The model under review builds one solid part; all positions refer to its coordinate system, in mm. Round coordinates to 2 decimals unless told otherwise and drop trailing zeros. Order: outer loops, then holes, each group sorted by start corner. A loop starts at its lowest first (then second) coordinate and runs counter-clockwise, first axis right, second up.
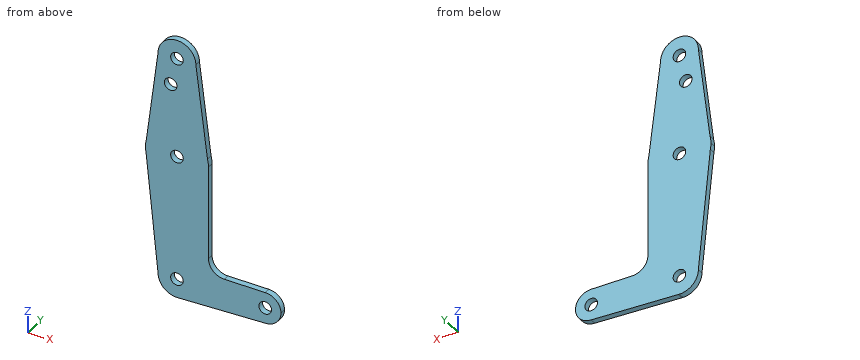
from build123d import *

# Parameters (mm, degrees)
F0_R     = 3.175
F1_DEPTH = 3.048


with BuildPart() as f1:
    # F0 (on Front) → F1 (new body)
    with BuildSketch(Plane.XZ):
        with BuildLine():
            ThreePointArc((-9.525, 114.3), (0, 104.775), (9.525, 114.3))
            ThreePointArc((9.525, 114.3), (0, 123.825), (-9.525, 114.3))
        make_face()
        with Locations((0, 114.3)):
            Circle(F0_R, mode=Mode.SUBTRACT)
        with BuildLine():
            Line((15.3865384615, 67.4076923077), (9.525, 114.3))
            ThreePointArc((9.525, 114.3), (0, 104.775), (-9.525, 114.3))
            Line((-9.525, 114.3), (-15.3865384615, 67.4076923077))
            ThreePointArc((-15.3865384615, 67.4076923077), (0, 79.375), (15.3865384615, 67.4076923077))
        make_face()
        with Locations((-3.175, 100.0252)):
            Circle(F0_R, mode=Mode.SUBTRACT)
        with BuildLine():
            Line((15.875, 63.5), (15.3865384615, 67.4076923077))
            ThreePointArc((15.3865384615, 67.4076923077), (0, 79.375), (-15.3865384615, 67.4076923077))
            Line((-15.3865384615, 67.4076923077), (-15.875, 63.5))
            Line((-15.875, 63.5), (-15.5606435644, 60.3564356436))
            ThreePointArc((-15.5606435644, 60.3564356436), (1.5796215395, 47.7037846054), (15.875, 63.5))
        make_face()
        with Locations((0, 63.5)):
            Circle(F0_R, mode=Mode.SUBTRACT)
        with BuildLine():
            ThreePointArc((15.875, 63.5), (15.7524112928, 65.4690514116), (15.3865384615, 67.4076923077))
            Line((15.3865384615, 67.4076923077), (15.875, 63.5))
        make_face()
        with BuildLine():
            Line((-15.875, 63.5), (-15.3865384615, 67.4076923077))
            ThreePointArc((-15.3865384615, 67.4076923077), (-15.7524112928, 65.4690514116), (-15.875, 63.5))
        make_face()
        with BuildLine():
            Line((15.875, 15.8877), (15.875, 63.5))
            ThreePointArc((15.875, 63.5), (1.5796215395, 47.7037846054), (-15.5606435644, 60.3564356436))
            Line((-15.5606435644, 60.3564356436), (-9.525, 0))
            ThreePointArc((-9.525, 0), (0, 9.525), (9.525, 0))
            ThreePointArc((9.525, 0), (6.9712901065, -6.4905114784), (0.6794904459, -9.5007324841))
            Line((0.6794904459, -9.5007324841), (44.45, -7.9375))
            ThreePointArc((44.45, -7.9375), (36.5125, 0), (44.45, 7.9375))
            Line((44.45, 7.9375), (23.8252, 7.9375))
            ThreePointArc((23.8252, 7.9375), (18.2035596682, 10.2660596682), (15.875, 15.8877))
        make_face()
        with BuildLine():
            Line((-15.5606435644, 60.3564356436), (-15.875, 63.5))
            ThreePointArc((-15.875, 63.5), (-15.7962153946, 61.9203784605), (-15.5606435644, 60.3564356436))
        make_face()
        with BuildLine():
            ThreePointArc((9.525, 0), (0, 9.525), (-9.525, 0))
            ThreePointArc((-9.525, 0), (-6.7351920908, -6.7351920908), (0, -9.525))
            Line((0, -9.525), (0.6794904459, -9.5007324841))
            ThreePointArc((0.6794904459, -9.5007324841), (6.9712901065, -6.4905114784), (9.525, 0))
        make_face()
        Circle(F0_R, mode=Mode.SUBTRACT)
        with BuildLine():
            Line((0.6794904459, -9.5007324841), (0, -9.525))
            ThreePointArc((0, -9.525), (0.3399618281, -9.5189311877), (0.6794904459, -9.5007324841))
        make_face()
        with BuildLine():
            ThreePointArc((52.3875, 0), (50.0626600757, 5.6126600757), (44.45, 7.9375))
            ThreePointArc((44.45, 7.9375), (36.5125, 0), (44.45, -7.9375))
            ThreePointArc((44.45, -7.9375), (50.0626600757, -5.6126600757), (52.3875, 0))
        make_face()
        with Locations((44.45, 0)):
            Circle(F0_R, mode=Mode.SUBTRACT)
    extrude(amount=F1_DEPTH)


solid = f1.part
(1) We need section A-A (y = -2.15). Count the separate pieces of the cut face and the enclosed holes in it, and give its area (3 significant figures).
(2) We need section B-B (x = 28). Give the boundary of the cut face in (y, z) (1 decimal), and give its area (3 significant figures).
(3) We need section C-C (z = 70). Give the boundary of the cut face in (x, y), and give its area (3 significant figures).
(4) Clearance check with flat-ended pins moving along their axes: P1, Ø4, axis at x = 0, z = 114.3, coming from the +Y side; P2, Ø1, axis at x = 2, y = -1.5, coming from the -Z side; P3, Ø1.5, axis at x = 34.5, y = -1.5, coming from the +Z side. State where each tip first meets the part, or that it passes through.
(5) To check wall thickness, follow L1, parallel to X at y = -0.6, z = 99; L2, parallel to Z at x = 46, y = -2.3; L3, parallel to X at y = -1.9, z = 73. State the ranges of each line that lie inside material, in increasing order.
Verdict:
1. separate pieces: 1
1. enclosed holes: 5
1. area: 3,890 mm2
2. outline: (-3, -8.5) - (0, -8.5) - (0, 7.9) - (-3, 7.9) - close
2. area: 50.2 mm2
3. outline: (-15.06, -3.05) - (15.06, -3.05) - (15.06, 0) - (-15.06, 0) - close
3. area: 91.8 mm2
4. P1: passes through
4. P2: stops at z = -9.47
4. P3: stops at z = 7.94
5. L1: x = -11.44 to -6.18, -0.17 to 11.44
5. L2: z = -7.78 to -2.77, 2.77 to 7.78
5. L3: x = -14.69 to 14.69
